Read the model definition and answer for the solid it produces. Units are mm, in the model's axes. Face numbers are marked on the shaded views. A direction names the side the tool comes from. Coordinates: 2 decimals unless noted, no trailing zeros. Write each loop counter-clockwise with the first axis right and the second up, starting at its lowest first coordinate (ties: lowest second). Pieces come first, ordered by that corner, then holes. Notation, with made-up numbers: (-21, -30.5) -> (-13, -30.5) arc R21 cw to (-13, -6.5) -> close; hole circle Ø9 at (-34.75, -2). An arc over 180 degrees is marked (long way). Use CSV: the item, a comma, the result in double quotes.
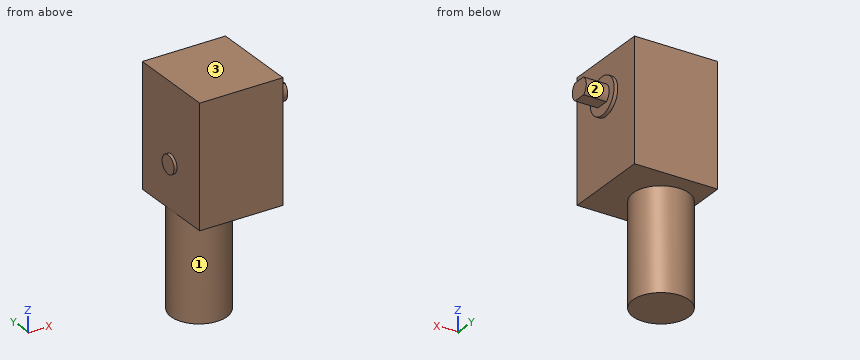
from build123d import *

# Parameters (mm, degrees)
SKETCH1_W             = 16.5
SKETCH1_H             = 12
BASE_DEPTH            = 11.3
SKETCH2_R             = 2.5
AXLE_BASE_DEPTH       = 0.5
AXLE_DEPTH            = 3.1
SKETCH4_R             = 3.8
WIRE_HOUSING_DEPTH    = 13.8
SKETCH5_R             = 1.25
RANDOM_ASS_BUMP_DEPTH = 0.4


with BuildPart() as part:
    # Sketch1 → Base (new body)
    with BuildSketch(Plane(origin=(0, 0, 0), x_dir=(0, 0, -1), z_dir=(1, 0, 0))):
        with Locations((3.05, 0)):
            Rectangle(SKETCH1_W, SKETCH1_H)
    extrude(amount=-BASE_DEPTH)

    # Sketch2 → Axle Base (add)
    with BuildSketch(Plane(origin=(0, 0, 0), x_dir=(0, 0, -1), z_dir=(1, 0, 0))):
        Circle(SKETCH2_R)
    extrude(amount=AXLE_BASE_DEPTH)

    # Sketch3 → Axle (add)
    with BuildSketch(Plane(origin=(0.5, 0, 0), x_dir=(0, 0, -1), z_dir=(1, 0, 0))):
        with BuildLine():
            Line((1.15, 0.899499861), (1.15, -0.899499861))
            ThreePointArc((1.15, -0.899499861), (0, -1.46), (-1.15, -0.899499861))
            Line((-1.15, -0.899499861), (-1.15, 0.899499861))
            ThreePointArc((-1.15, 0.899499861), (0, 1.46), (1.15, 0.899499861))
        make_face()
    extrude(amount=AXLE_DEPTH)

    # Sketch4 → Wire Housing (add)
    with BuildSketch(Plane(origin=(0, 0, -11.3), x_dir=(-1, 0, 0), z_dir=(0, 0, -1))):
        with Locations((7.5, 0)):
            Circle(SKETCH4_R)
    extrude(amount=WIRE_HOUSING_DEPTH)

    # Sketch5 → Random-ass Bump (add)
    with BuildSketch(Plane.ZY.offset(11.3)):
        with Locations(Location((-5.3, 0, 0), (0, 0, 180))):
            Circle(SKETCH5_R)
    extrude(amount=RANDOM_ASS_BUMP_DEPTH)


solid = part.part
1. A cutting plane is placed at B-B (z = 0). Give the vertices of the cut face in (x, y).
Solutions:
outline,"(-11.3, -6) -> (0, -6) -> (0, -2.5) -> (0.5, -2.5) -> (0.5, -1.46) -> (3.6, -1.46) -> (3.6, 1.46) -> (0.5, 1.46) -> (0.5, 2.5) -> (0, 2.5) -> (0, 6) -> (-11.3, 6) -> close"
2. Each of these flat-tipped pins is pushed along its axis until it touches: pin 1 Ø5 at (y, z) = (-3.5, -18.5) entering from -X; pin 2 Ø5 at (x, z) = (-8.5, -15.5) entering from +Y; pin 3 Ø2 at (y, z) = (1.5, 1.5) entering from -X. Where does it stop, or does it pass through?
Solutions:
pin 1,"stops at x = -11.17"
pin 2,"stops at y = 3.8"
pin 3,"stops at x = -11.3"
3. A cutting plane is placed at D-D (x = -3.25). Give the vertices of the cut face in (y, z).
Solutions:
outline,"(-6, -11.3) -> (6, -11.3) -> (6, 5.2) -> (-6, 5.2) -> close"
4. Find the intervals of material crossed by line 1 along Z through (x, y) = (-2.25, 2.5); line 2 along X through (y, z) = (1.5, -1); line 3 along X through (y, z) = (-1.25, 0), in increasing order.
Solutions:
line 1,"z = -11.3 to 5.2"
line 2,"x = -11.3 to 0.5"
line 3,"x = -11.3 to 3.6"
5. A cutting plane is placed at C-C (y = 3). Give the vertices of the cut face in (x, z), and give its area (3 significant figures).
Solutions:
outline,"(-11.3, -11.3) -> (-9.83, -11.3) -> (-9.83, -25.1) -> (-5.17, -25.1) -> (-5.17, -11.3) -> (0, -11.3) -> (0, 5.2) -> (-11.3, 5.2) -> close"
area,"251 mm^2"
6. A tool of negligible diameter and unlimited length cuts with its end or side. For the marked faces 1, 2 and 3, from which of +Z, -Z, +X, -X, +Y, -Y can it reach the whole face along a straight path? Write none if from no direction.
Solutions:
face 1,"-Z"
face 2,"+X, +Y"
face 3,"+Z, +X, -X, +Y, -Y"
7. A cutting plane is placed at A-A (x = -7.5). Give the vertices of the cut face in (y, z).
Solutions:
outline,"(-6, -11.3) -> (-3.8, -11.3) -> (-3.8, -25.1) -> (3.8, -25.1) -> (3.8, -11.3) -> (6, -11.3) -> (6, 5.2) -> (-6, 5.2) -> close"
